Can you work these out from the model? Positions are in its coordinate system, mm. Face numbers are marked on the shaded views. A direction names the side the tool comes from. Round coordinates to 2 decimals unless told otherwise and drop trailing zeros. Order: outer loops, then holes, each group sorted by start corner. A loop starts at its lowest first (then second) coordinate and runs counter-clockwise, first axis right, second up.
Q1. If we section it at C-C (z = -6.75): Count the separate pieces of the cut face and the enclosed holes in it, plus the area to 3 significant figures.
Q2. If I drill on line 1 (Y direction, x = 0, z = -1.25); line 2 (Y direction, x = 22.5, z = -5.5) (3 decimals); line 3 (Y direction, x = -14.5, z = -6.25) (3 decimals), over which ranges is the centre line in solid material (lowest first)?
Q3. Will these pins go through, and if not, where does the flat tip stop? P1, Ø6, axis at x = 39.975, y = 63, coming from the +Z side; P2, Ø8, axis at x = 2, z = -4, coming from the +Y side; P3, Ø12, axis at x = 32, y = -12.5, coming from the -Z side (3 decimals).
Q4. If we section it at D-D (x = 30.5): Please give me the cut outline in (y, z) (3 decimals).
Q5. We'd pull the mould along Y, two halves only. Please class the marked faces 3, 4 and 5: pulls with the +Y half, pulls with the -Y half, needs draft (parallel to the pull), parting line crosses it, or undercut.
Q6. If we section it at A-A (x = -4): Please give me the cut outline in (y, z) (3 decimals).
Q7. For the marked faces 1 and 2, which set-ups out of +Z, -Z, +X, -X, +Y, -Y let a thin tool reach every point of the face, with its end or its side?
Q8. If we section it at B-B (y = 63): Please give me the cut outline in (x, z) (3 decimals), plus the area to 3 significant figures.
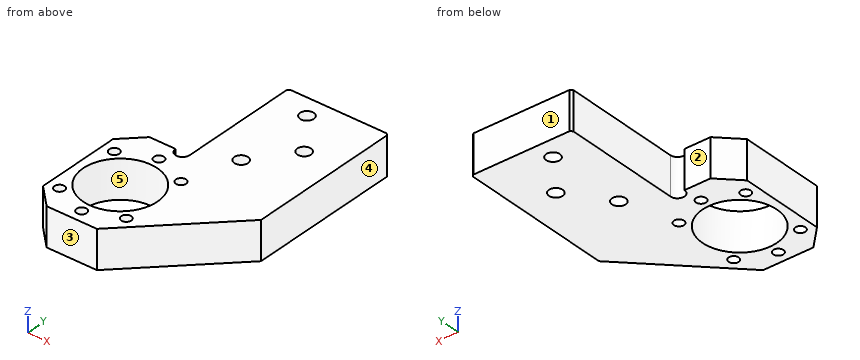
from build123d import *

# Parameters (mm, degrees)
SKETCH1_R              = 18.5
BOSS_EXTRUDE1_DEPTH    = 9.525
M8X1_25_TAPPED_HOLE1_D = 6.8
TAPPED_HOLE0_D         = 5
CHAMFER1_SIZE          = 1


with BuildPart() as part:
    # Sketch1 → Boss-Extrude1 (new, symmetric)
    with BuildSketch(Plane.XY):
        with BuildLine():
            Line((0.475, 33), (-12.525, 33))
            Line((-12.525, 33), (-22.525, 23))
            Line((-22.525, 23), (-22.525, -19.5))
            Line((-22.525, -19.5), (-12.525, -29.5))
            Line((-12.525, -29.5), (12.525, -29.5))
            Line((12.525, -29.5), (57.475, 15.45))
            Line((57.475, 15.45), (57.475, 93))
            Line((57.475, 93), (7.475, 93))
            Line((7.475, 93), (7.475, 33))
            ThreePointArc((7.475, 33), (3.975, 29.5), (0.475, 33))
        make_face()
        with Locations(Location((0, 0, 0), (0, 0, 180))):
            Circle(SKETCH1_R, mode=Mode.SUBTRACT)
    extrude(amount=BOSS_EXTRUDE1_DEPTH, both=True)

    # M8x1.25 Tapped Hole1 (through all)
    with Locations(Plane.XY.offset(9.525)):
        with Locations((24.975, 43), (39.975, 63), (24.975, 83)):
            Hole(M8X1_25_TAPPED_HOLE1_D / 2)

    # Tapped Hole0 (through all)
    with Locations(Plane.XY.offset(9.525)):
        with Locations((0, 23.5), (-16.617009358, 16.617009358), (16.617009358, 16.617009358), (16.617009358, -16.617009358), (0, -23.5), (-16.617009358, -16.617009358)):
            Hole(TAPPED_HOLE0_D / 2)

    # Chamfer1
    chamfer1_edges = [part.edges().sort_by_distance(p)[0] for p in [
        (7.475, 93, 0),
        (57.475, 93, 0),
    ]]
    chamfer(chamfer1_edges, length=CHAMFER1_SIZE)


solid = part.part
Solution:
1. separate pieces: 1
1. enclosed holes: 10
1. area: 5,570 mm2
2. line 1: y = -29.5 to -26, -21 to -18.5, 18.5 to 21, 26 to 33
2. line 2: y = -19.525 to 40.669, 45.331 to 80.669, 85.331 to 93
2. line 3: y = -27.525 to -17.947, -15.287 to -11.489, 11.489 to 15.287, 17.947 to 31.025
3. P1: passes through
3. P2: stops at y = 33
3. P3: stops at z = -9.525
4. outline: (-11.525, -9.525) - (93, -9.525) - (93, 9.525) - (-11.525, 9.525) - close
5. face 3: pulls with the -Y half
5. face 4: needs draft
5. face 5: undercut
6. outline: (-29.5, -9.525) - (-18.062, -9.525) - (-18.062, 9.525) - (-29.5, 9.525) - close; (18.062, -9.525) - (33, -9.525) - (33, 9.525) - (18.062, 9.525) - close
7. face 1: +Z, -Z, +X, -X, +Y
7. face 2: +Z, -Z, -X, +Y
8. outline: (7.475, -9.525) - (36.575, -9.525) - (36.575, 9.525) - (7.475, 9.525) - close; (43.375, -9.525) - (57.475, -9.525) - (57.475, 9.525) - (43.375, 9.525) - close
8. area: 823 mm2
